Answer from the drawing. Dimensions are ordinates in mm from the lowest x, y and z of the part. Round coordinates to 2 decimals unless told otherwise and drop trailing zeros. Order: outer loops, then holes, each group sorted by start corner. A loop starts at its lowest first (then second) coordinate and runs counter-clockwise, first axis right, second up. Notation, with made-up numbers: M 13,44 L 29,44 A13 ccw 29,66 Z; hole C 10,16.25 d5. An arc over 180 degrees is marked long. Use one line per item in the form item = value. Start each with the question number.
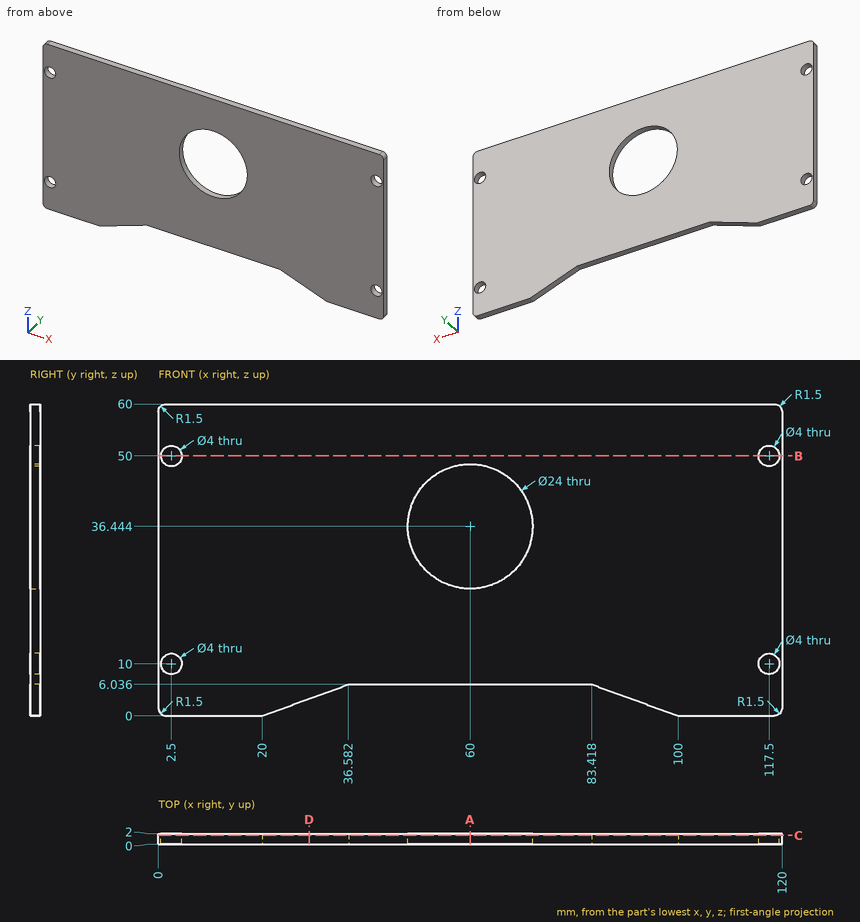
Item 1: Given P1, Ø3.5, axis at x = 2.5, z = 50, coming from the +Y side, flat-ended and moving along its own axis, determine where the tip first touches the part or whether it passes through.
Item 2: Section B-B (z = 50) is taken. Write down the section's boundary in (x, y).
Item 3: Section C-C (y = 1.7) is taken. Write down the section's boundary in (x, z) (1 decimal).
Item 4: Section D-D (x = 29) is taken. Write down the section's boundary in (y, z) (1 decimal).
Item 5: Section A-A (x = 60) is taken. Write down the section's boundary in (y, z) (1 decimal).
Item 6: Find the intervals of material crossed by L1, parallel to X at y = 1.1, z = 10; L2, parallel to X at y = 1, z = 43; L3, parallel to Z at x = 61, y = 0.25 (1 decimal), in increasing order. Write a range as [from, to].
The answers:
q1.P1 = through
q2.outline = M 0,0 L 0.5,0 L 0.5,2 L 0,2 Z; M 4.5,0 L 115.5,0 L 115.5,2 L 4.5,2 Z; M 119.5,0 L 120,0 L 120,2 L 119.5,2 Z
q3.outline = M 0,1.5 A1.5 ccw 1.5,0 L 20,0 L 36.6,6 L 83.4,6 L 100,0 L 118.5,0 A1.5 ccw 120,1.5 L 120,58.5 A1.5 ccw 118.5,60 L 1.5,60 A1.5 ccw 0,58.5 Z; hole C 2.5,10 d4; hole C 2.5,50 d4; hole C 60,36.4 d24; hole C 117.5,10 d4; hole C 117.5,50 d4
q4.outline = M 0,3.3 L 2,3.3 L 2,60 L 0,60 Z
q5.outline = M 0,6 L 2,6 L 2,24.4 L 0,24.4 Z; M 0,48.4 L 2,48.4 L 2,60 L 0,60 Z
q6.L1 = [0, 0.5], [4.5, 115.5], [119.5, 120]
q6.L2 = [0, 49.95], [70.05, 120]
q6.L3 = [6, 24.5], [48.4, 60]
